Read the model definition and answer for the solid it produces. Units are mm, in the model's axes. A direction names the side the tool comes from. Round coordinates to 2 decimals unless told otherwise and drop trailing zeros. Write each question's results on one line, items separated by ' | '.
from build123d import *

# Parameters (mm, degrees)
F0_R     = 15.9252412
F1_DEPTH = 25.4
F2_R     = 12.69999
F5_DEPTH = 3.81


# Not quite as in the source:
# - a fillet or chamfer is up to 0.001 mm smaller than in the source, because OpenCascade refuses the exact size


with BuildPart() as f1:
    # F0 (on Top) → F1 (new body)
    with BuildSketch(Plane.XY):
        with Locations((-33.0793492307, 17.5561513754)):
            Circle(F0_R)
    extrude(amount=F1_DEPTH)

    # F2 (radius 12.7 in the source; OpenCascade refuses exactly that, so slightly less here)
    f2_edges = [f1.edges().sort_by_distance(p)[0] for p in [
        (-49.00459, 17.556151, 25.4),
        (-49.00459, 17.556151, 0),
    ]]
    fillet(f2_edges, radius=F2_R)

    # F4 (on offset) → F5 (join)
    with BuildSketch(Plane.XZ.offset(-4.318)):
        with BuildLine():
            Line((-29.0207639337, 14.9749675766), (-27.8811603785, 16.3556560874))
            ThreePointArc((-27.8811603785, 16.3556560874), (-28.0885315249, 16.9271168776), (-28.695197776, 16.9661846012))
            Line((-28.695197776, 16.9661846012), (-29.4164977968, 15.9463118762))
            ThreePointArc((-29.4164977968, 15.9463118762), (-35.315728181, 15.6618586245), (-36.2196562996, 9.8253573836))
            ThreePointArc((-36.2196562996, 9.8253573836), (-36.219121003, 9.824445743), (-36.2185855, 9.8235342236))
            Line((-36.2185855, 9.8235342236), (-37.5962145627, 8.0000562593))
            Line((-37.5962145627, 8.0000562593), (-34.392606223, 8.0947948317))
            ThreePointArc((-34.392606223, 8.0947948317), (-34.3897808352, 8.0934481012), (-34.3869543323, 8.0921037126))
            ThreePointArc((-34.3869543323, 8.0921037126), (-30.5469478577, 8.4474204279), (-29.0207639337, 11.9889825583))
            ThreePointArc((-29.0207639337, 11.9889825583), (-30.3891986708, 14.106652787), (-32.9061411321, 14.2554529011))
            ThreePointArc((-32.9061411321, 14.2554529011), (-34.717169495, 12.4733526926), (-34.0933389962, 10.0103178993))
            ThreePointArc((-34.0933389962, 10.0103178993), (-31.6624363369, 9.8503464108), (-30.4957684129, 11.9889825583))
            ThreePointArc((-30.4957684129, 11.9889825583), (-31.4214059538, 12.9964876797), (-32.7661586101, 12.7444723621))
            ThreePointArc((-32.7661586101, 12.7444723621), (-33.4490909653, 11.6472132504), (-32.7661586101, 10.5499541387))
            ThreePointArc((-32.7661586101, 10.5499541387), (-31.7571819842, 10.9231691425), (-31.6110141575, 11.9889825583))
            ThreePointArc((-31.6110141575, 11.9889825583), (-31.7935886004, 12.08811911), (-31.8988275295, 11.9089927555))
            ThreePointArc((-31.8988275295, 11.9089927555), (-31.9495376202, 11.212409195), (-32.6134748757, 10.9956432134))
            ThreePointArc((-32.6134748757, 10.9956432134), (-33.1081520423, 11.7169185542), (-32.6134748757, 12.4381938949))
            ThreePointArc((-32.6134748757, 12.4381938949), (-31.714287938, 12.6534772255), (-31.0713797808, 11.9889825583))
            ThreePointArc((-31.0713797808, 11.9889825583), (-31.8928919194, 10.1846295294), (-33.841509372, 10.5499541387))
            ThreePointArc((-33.841509372, 10.5499541387), (-34.1573684854, 12.4434120609), (-32.7527012902, 13.7517927215))
            ThreePointArc((-32.7527012902, 13.7517927215), (-30.7985222002, 13.6359080863), (-29.7402776778, 11.9889825583))
            ThreePointArc((-29.7402776778, 11.9889825583), (-31.4290089637, 8.6919853613), (-35.1006612182, 9.182875976))
            ThreePointArc((-35.1006612182, 9.182875976), (-34.7993943786, 14.9536870948), (-29.0207639337, 14.9749675766))
        make_face()
        with BuildLine():
            Line((-36.8709181573, 8.4690021479), (-36.0997095704, 9.489800781))
            ThreePointArc((-36.0997095704, 9.489800781), (-35.713386033, 8.8381304316), (-35.107601434, 8.383218199))
            Line((-35.107601434, 8.383218199), (-36.8709181573, 8.4690021479))
        make_face(mode=Mode.SUBTRACT)
    extrude(amount=F5_DEPTH)


solid = f1.part
Item 1: Straight lines are drawn through the part: line 1 (X direction, y = 12, z = 12.75); line 2 (Y direction, x = -25, z = 13); line 3 (Z direction, x = -41, y = 25). For each, find the intervals that lie inside material, in ascending order.
Outcome:
line 1: x = -48 to -18.15 | line 2: y = 3.84 to 31.28 | line 3: z = 2.56 to 22.84
Item 2: For faces 1 (the face through (-29.051, 1.779, 16.463)), 2 (the face through (-30.82, 1.1, 13.65)), 3 (the face through (-28.459, 1.523, 15.656)), 4 (the face through (-33, 0.508, 11)), determine the directions among +Z, -Z, +X, -X, +Y, -Y from which every point of the face is accessible in a straight line to the end or side of a thin tool.
Outcome:
face 1: +Z, -Y | face 2: -Y | face 3: +X, -Y | face 4: +Z, -Z, +X, -X, -Y
Item 3: The mould has two halves that part along X. Classify faces 5 (the face through (-31.943, 1.146, 11.221)), 6 (the face through (-36.9, 1.58, 8.92)), 7 (the face through (-33, 18, 25.4)): pulls with the +X half, pulls with the -X half, needs draft (parallel to the pull), parting line crosses it, or undercut.
Outcome:
face 5: undercut | face 6: pulls with the -X half | face 7: needs draft
Item 4: Flat-ended cylindrical pins translate along their axes: pin 1 (2 mm diameter, centred on y = 27, z = 3.5, fed in from -X); pin 2 (6 mm diameter, centred on x = -25.5, z = 5, fed in from -Y); pin 3 (1 mm diameter, centred on x = -40, z = 4.5, fed in from -Y). Find the tip coordinate at first contact, or state that the pin passes through.
Outcome:
pin 1: stops at x = -42.26 | pin 2: stops at y = 3.96 | pin 3: stops at y = 6.08
